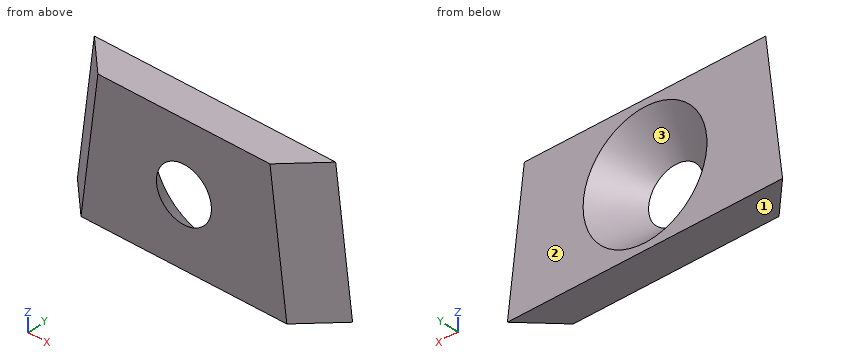
```python
from build123d import *

# Parameters (mm, degrees)
F1_DEPTH = 3.175
F2_SIZE  = 3.17499
F3_R     = 2.54
F4_DEPTH = 25.4
F5_SIZE  = 3.17499


# Not quite as in the source:
# - a fillet or chamfer is up to 0.001 mm smaller than in the source, because OpenCascade refuses the exact size


with BuildPart() as f1:
    # F0 (on Front) → F1 (new body)
    with BuildSketch(Plane.XZ):
        Polygon((1.5593639235, 12.7), (0, 0), (25.4, 0), (23.8406360765, 12.7), align=None)
    extrude(amount=F1_DEPTH)

    # F2 (size 3.175 in the source; OpenCascade refuses exactly that, so slightly less here)
    f2_edges = [f1.edges().sort_by_distance(p)[0] for p in [
        (24.620318, -3.175, 6.35),
        (0.779682, -3.175, 6.35),
    ]]
    chamfer(f2_edges, length=F2_SIZE)

    # F3 (on face) → F4 (cut)
    with BuildSketch(Plane.XZ.offset(3.175)):
        with Locations((12.7, 6.35)):
            Circle(F3_R)
    extrude(amount=-F4_DEPTH, mode=Mode.SUBTRACT)

    # F5 (size 3.175 in the source; OpenCascade refuses exactly that, so slightly less here)
    f5_edges = [f1.edges().sort_by_distance(p)[0] for p in [
        (10.16, 0, 6.35),
    ]]
    chamfer(f5_edges, length=F5_SIZE)


solid = f1.part
```
Source: CAD feature listing. Evaluate the final solid. Frame: model axes, mm. Face numbers are marked on the shaded views. Round coordinates to 2 decimals unless told otherwise and drop trailing zeros. Order: outer loops, then holes, each group sorted by start corner. A loop starts at its lowest first (then second) coordinate and runs counter-clockwise, first axis right, second up. Notation, with made-up numbers: (49.25, 27) -> (68.25, 27) arc R20 ccw to (68.25, 46) -> close; hole circle Ø8 at (48.5, 64). An arc over 180 degrees is marked (long way). One line per item, written item: value. Start each with the question number.
Q1. Section query D-D (y = -2.9). Return the cut outline in (x, z) (3 decimals), plus the area to 3 significant figures.
Q2. Section query C-C (y = -0.9). Return the cut outline in (x, z).
Q3. Material intervals for probe 1 along X at (y, z) = (-1.5, 9); probe 2 along X at (y, z) = (-0.5, 8.25); probe 3 along Y at (x, z) = (18.25, 5) (3 decimals), sorted ascending.
Q4. Pin query (flat end, axial travel): pin 1 (1.5 mm diameter, centred on y = -2.5, z = 1.5, fed in from -X); pin 2 (1 mm diameter, centred on x = 13.5, z = 1.5, fed in from +Y); pin 3 (1.5 mm diameter, centred on y = -1.5, z = 6.5, fed in from +X). Return the tip coordinate at first contact, or that it passes through.
Q5. Draft query along Z for the marked faces 1, 2 and 3. Return one class per face: pulls with the +Z half, pulls with the -Z half, needs draft (parallel to the pull), parting line crosses it, or undercut.
Findings below:
1. outline: (2.922, 0) -> (22.478, 0) -> (20.919, 12.7) -> (4.481, 12.7) -> close; hole circle Ø5.63 at (12.7, 6.35)
1. area: 204 mm²
2. outline: (0.91, 0) -> (24.49, 0) -> (22.93, 12.7) -> (2.47, 12.7) -> close; hole circle Ø9.63 at (12.7, 6.35)
3. probe 1: 2.62 to 9.42, 15.98 to 22.78
3. probe 2: 1.52 to 7.84, 17.56 to 23.88
3. probe 3: -3.175 to -0.003
4. pin 1: x = 1.94
4. pin 2: y = -0.3
4. pin 3: x = 23.85
5. face 1: pulls with the -Z half
5. face 2: needs draft
5. face 3: undercut
